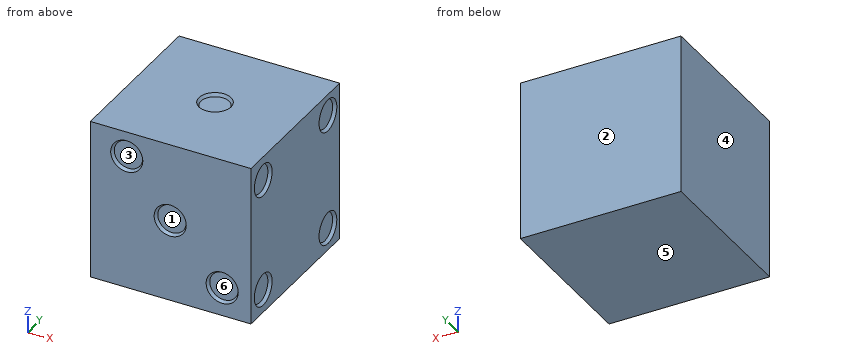
from build123d import *

# Parameters (mm, degrees)
F0_W     = 25.4
F0_H     = 25.4
F1_DEPTH = 25.4
F2_R     = 2.54
F3_DEPTH = 0.508
F3_TAPER = 30
F4_R     = 2.54
F5_DEPTH = 0.508
F5_TAPER = 30
F6_R     = 2.54
F7_DEPTH = 0.508
F7_TAPER = 30


with BuildPart() as f1:
    # F0 (on Top) → F1 (new body)
    with BuildSketch(Plane.XY):
        Rectangle(F0_W, F0_H)
    extrude(amount=F1_DEPTH)

    # F2 (on face) → F3 (cut)
    with BuildSketch(Plane.XY.offset(25.4)):
        Circle(F2_R)
    extrude(amount=-F3_DEPTH, taper=F3_TAPER, mode=Mode.SUBTRACT)

    # F4 (on face) → F5 (cut)
    with BuildSketch(Plane.XZ.offset(12.7)):
        with Locations((-6.9411581597, 21.445404164)):
            Circle(F4_R)
        with Locations((-0.069737803, 13.023638883)):
            Circle(F4_R)
        with Locations((8.1521372762, 4.5340581903)):
            Circle(F4_R)
    extrude(amount=-F5_DEPTH, taper=F5_TAPER, mode=Mode.SUBTRACT)

    # F6 (on face) → F7 (cut)
    with BuildSketch(Plane.YZ.offset(12.7)):
        with Locations((-9.188728149, 21.5874935842)):
            Circle(F6_R)
        with Locations((9.3399413093, 22.001354984)):
            Circle(F6_R)
        with Locations((9.3340705111, 3.5717650137)):
            Circle(F6_R)
        with Locations((-9.1927518238, 3.6942041952)):
            Circle(F6_R)
    extrude(amount=-F7_DEPTH, taper=F7_TAPER, mode=Mode.SUBTRACT)


solid = f1.part
Work out the finished part from the listing and answer in its coordinate system (mm). Face numbers are marked on the shaded views. A direction names the side the tool comes from. Round coordinates to 2 decimals unless told otherwise and drop trailing zeros. One line per item, written item: value.
Q1. Straight lines are drawn through the part: probe 1 along X at (y, z) = (-8.5, 21); probe 2 along Z at (x, y) = (0.5, 1); probe 3 along Y at (x, z) = (8, 7). For each, find the intervals that lie inside material, in ascending order.
Check values:
probe 1: -12.7 to 12.19
probe 2: 0 to 24.89
probe 3: -12.58 to 12.7
Q2. Each of these flat-tipped pins is pushed along its axis until it touches: pin 1 Ø2 at (y, z) = (-10, 3) entering from +X; pin 2 Ø1.3 at (x, y) = (0, 0.5) entering from +Z; pin 3 Ø2 at (x, z) = (0.5, 14) entering from -Y. Where does it stop, or does it pass through?
Check values:
pin 1: x = 12.19
pin 2: z = 24.89
pin 3: y = -12.19
Q3. For the marked faces 1 and 2, determine the directions among +Z, -Z, +X, -X, +Y, -Y from which every point of the face is accessible in a straight line to the end or side of a thin tool.
Check values:
face 1: -Y
face 2: +Z, -Z, +X, -X, +Y
Q4. The mould has two halves that part along Z. Classify the marked faces 3, 4, 5 and 6: +Z half, -Z half, draft (parallel to the pull), parting line (faces both ways), or undercut.
Check values:
face 3: undercut
face 4: draft
face 5: -Z half
face 6: undercut
